Source: CAD feature listing. Evaluate the final solid. Frame: model axes, mm. Face numbers are marked on the shaded views. A direction names the side the tool comes from. Give positions to 0.01 mm unless a question says otherwise; leave off trailing zeros. Loops run counter-clockwise (first coordinate to the right, second up) from the corner with the lowest first, then second, coordinate; pieces in that order, holes last.
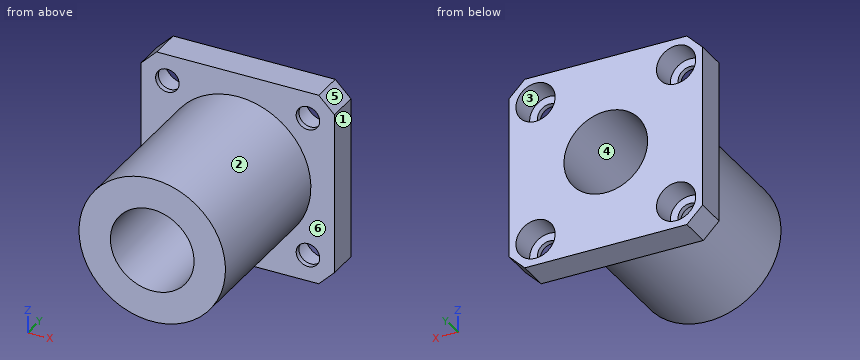
```python
from build123d import *

# Parameters (mm, degrees)
SKETCH_1_R                   = 14
SKETCH_1_R_2                 = 8
EXTRUDE_1_DEPTH              = 37
EXTRUDE_START                = -6
SKETCH_2_W                   = 37
SKETCH_2_H                   = 37
SKETCH_2_R                   = 8
EXTRUDE_2_DEPTH              = 6
HOLE_WIZARD_M3_1_D           = 4.5
HOLE_WIZARD_M3_1_CBORE_D     = 7.5
HOLE_WIZARD_M3_1_CBORE_DEPTH = 5
CHAMFER_1_SIZE               = 3


with BuildPart() as part:
    # 草图1 → 凸台-拉伸1 (new body)
    with BuildSketch(Plane(origin=(0, 0, 0), x_dir=(1, 0, 0), z_dir=(0, 1, 0))):
        with Locations(Location((0, 0, 0), (0, 0, 270))):
            Circle(SKETCH_1_R)
        with Locations(Location((0, 0, 0), (0, 0, 270))):
            Circle(SKETCH_1_R_2, mode=Mode.SUBTRACT)
    extrude(amount=EXTRUDE_1_DEPTH)

    # 草图2 → 凸台-拉伸2 (add)
    with BuildSketch(Plane(origin=(0, 37, 0), x_dir=(1, 0, 0), z_dir=(0, 1, 0)).offset(EXTRUDE_START)):
        Rectangle(SKETCH_2_W, SKETCH_2_H)
        with Locations(Location((0, 0, 0), (0, 0, 270))):
            Circle(SKETCH_2_R, mode=Mode.SUBTRACT)
    extrude(amount=EXTRUDE_2_DEPTH)

    # M3 六角头螺栓的柱形沉头孔1 (through all)
    with Locations(Plane(origin=(0, 37, 0), x_dir=(-1, 0, 0), z_dir=(0, 1, 0))):
        with Locations((-13.435028843, 13.435028843), (13.435028843, 13.435028843), (13.435028843, -13.435028843), (-13.435028843, -13.435028843)):
            CounterBoreHole(HOLE_WIZARD_M3_1_D / 2, HOLE_WIZARD_M3_1_CBORE_D / 2, HOLE_WIZARD_M3_1_CBORE_DEPTH)

    # 倒角1
    chamfer_1_edges = [part.edges().sort_by_distance(p)[0] for p in [
        (-18.5, 34, 18.5),
        (-18.5, 34, -18.5),
        (18.5, 34, -18.5),
        (18.5, 34, 18.5),
    ]]
    chamfer(chamfer_1_edges, length=CHAMFER_1_SIZE)


solid = part.part
```
(1) Section B-B, the plane x = 0. Return the cut outline in (y, z), then the cut area to 3 significant figures.
A:
outline: (0, -14) - (31, -14) - (31, -18.5) - (37, -18.5) - (37, -8) - (0, -8) - close; (0, 8) - (37, 8) - (37, 18.5) - (31, 18.5) - (31, 14) - (0, 14) - close
area: 498 mm2
(2) Section D-D, the plane y = 23. Return the cut outline in (x, z), then the cut area to 3 significant figures.
A:
outline: circle Ø28 at (0, 0); hole circle Ø16 at (0, 0)
area: 415 mm2
(3) Ray query, line 1 along Z through (x, y) = (12, 32.5); line 2 along Y through (x, z) = (2, -14); line 3 along X through (y, z) = (14, 0). Return the intervals inside material, ascending.
A:
line 1: z = -18.5 to -16.9, -9.97 to 9.97, 16.9 to 18.5
line 2: y = 31 to 37
line 3: x = -14 to -8, 8 to 14
(4) First-contact query: pin 1 (12 mm diameter, centred on x = 0, y = 21.5, fed in from -Z); pin 2 (4 mm diameter, centred on x = 13.44, z = 13.44, fed in from -Y); pin 3 (5 mm diameter, centred on x = -13.44, z = 13.44, fed in from +Y); pin 4 (2 mm diameter, centred on y = 24.5, z = 0.5, fed in from +X). Flat tips, straight axial feed; report the tip coordinate or a pass-through.
A:
pin 1: stops at z = -14
pin 2: passes through
pin 3: stops at y = 32
pin 4: stops at x = 14
(5) Section A-A, the plane z = 0. Return the cut outline in (x, y), then the cut area to 3 significant figures.
A:
outline: (-18.5, 31) - (-14, 31) - (-14, 0) - (-8, 0) - (-8, 37) - (-18.5, 37) - close; (8, 0) - (14, 0) - (14, 31) - (18.5, 31) - (18.5, 37) - (8, 37) - close
area: 498 mm2
(6) Section C-C, the plane y = 33. Return the cut outline in (x, z).
A:
outline: (-18.5, -15.5) - (-15.5, -18.5) - (15.5, -18.5) - (18.5, -15.5) - (18.5, 15.5) - (15.5, 18.5) - (-15.5, 18.5) - (-18.5, 15.5) - close; hole circle Ø7.5 at (-13.44, -13.44); hole circle Ø7.5 at (-13.44, 13.44); hole circle Ø16 at (0, 0); hole circle Ø7.5 at (13.44, -13.44); hole circle Ø7.5 at (13.44, 13.44)
(7) Mould query, pull axis X, two halves, no side actions, for the marked faces 4, 5 and 6. Classes: pulls with the +X half, pulls with the -X half, needs draft (parallel to the pull), parting line crosses it, or undercut.
A:
face 4: undercut
face 5: pulls with the +X half
face 6: needs draft
(8) Reachability of the marked faces 1, 2 and 3 from +Z, -Z, +X, -X, +Y, -Y: full face, straight path, thin tool, end or side. Return the list, or none.
A:
face 1: +Z, -Z, +X, +Y, -Y
face 2: -Y
face 3: +Y
